from build123d import *

# Parameters (mm, degrees)
EXTRUDE_1_DEPTH            = 10
SKETCH_3_W                 = 250
SKETCH_3_H                 = 25
EXTRUDE_3_DEPTH            = 15
SKETCH_4_W                 = 275.84447974
SKETCH_4_H                 = 25
EXTRUDE_4_DEPTH            = 15
SKETCH_10_W                = 250
SKETCH_10_H                = 30
EXTRUDE_5_DEPTH            = 15
SKETCH_11_W                = 275.84447974
SKETCH_11_H                = 30
EXTRUDE_6_DEPTH            = 15
HOLE_WIZARD_M5_1_D         = 4.2
HOLE_WIZARD_M5_1_DEPTH     = 15
PATTERN_LINEAR_1_COUNT     = 5
PATTERN_LINEAR_1_PITCH     = 50
MIRROR_1_COPY_1_D          = 4.2
MIRROR_1_COPY_1_DEPTH      = 15
MIRROR_1_COPY_2_D          = 4.2
MIRROR_1_COPY_2_DEPTH      = 15
MIRROR_1_COPY_3_D          = 4.2
MIRROR_1_COPY_3_DEPTH      = 15
MIRROR_1_COPY_4_D          = 4.2
MIRROR_1_COPY_4_DEPTH      = 15
HOLE_WIZARD_M5_2_D         = 4.2
PATTERN_START              = 218.95644092
PATTERN_LINEAR_2_OUTLINE_R = 2.1
PATTERN_LINEAR_2_DEPTH     = 15
HOLE_WIZARD_M5_3_D         = 4.2
PATTERN_LINEAR_3_OUTLINE_R = 2.1
PATTERN_LINEAR_3_DEPTH     = 15


# Read off the part's stored shape, not the designer's step: 阵列(线性)2, 阵列(线性)3
with BuildPart() as part:
    # 草图1 → 凸台-拉伸1 (new body)
    with BuildSketch(Plane.XY):
        Polygon((-125.313283208, 0), (124.686716792, 0), (124.686716792, 200), (-125.313283208, 316.576914539), align=None)
        Polygon((-110.313283208, 24.592855818), (-110.313283208, 280.944896886), (14.053831361, 123.772207379), (-107.63654934, 26.72747742), align=None, mode=Mode.SUBTRACT)
        Polygon((23.361623829, 112.009204107), (100.122763689, 15), (-98.284208811, 15), align=None, mode=Mode.SUBTRACT)
        Polygon((109.686716792, 180.85109027), (109.686716792, 27.086733996), (35.089185859, 121.36161211), align=None, mode=Mode.SUBTRACT)
        Polygon((-95.156980934, 285.964131062), (102.096111819, 193.983503317), (100.334376264, 192.57856769), (25.781393391, 133.124615382), align=None, mode=Mode.SUBTRACT)
    extrude(amount=EXTRUDE_1_DEPTH)

    # 草图3 → 凸台-拉伸3 (add)
    with BuildSketch(Plane.XZ):
        with Locations((-0.313283208, 5)):
            Rectangle(SKETCH_3_W, SKETCH_3_H)
    extrude(amount=-EXTRUDE_3_DEPTH)

    # 草图4 → 凸台-拉伸4 (add)
    with BuildSketch(Plane(origin=(98.874264385, 212.036544233, 0), x_dir=(0.9063077870366497, -0.4226182617407002, 0), z_dir=(0.42261826174070016, 0.9063077870366496, 0))):
        with Locations((-109.44134985, -5)):
            Rectangle(SKETCH_4_W, SKETCH_4_H)
    extrude(amount=-EXTRUDE_4_DEPTH)

    # 草图10 → 凸台-拉伸5 (add)
    with BuildSketch(Plane.XZ):
        with Locations((-0.313283208, 32.5)):
            Rectangle(SKETCH_10_W, SKETCH_10_H)
        with Locations((-0.313283208, -22.5)):
            Rectangle(SKETCH_10_W, SKETCH_10_H)
    extrude(amount=-EXTRUDE_5_DEPTH)

    # 草图11 → 凸台-拉伸6 (add)
    with BuildSketch(Plane(origin=(98.874264385, 212.036544233, 0), x_dir=(0.9063077870366497, -0.4226182617407002, 0), z_dir=(0.42261826174070016, 0.9063077870366496, 0))):
        with Locations((-109.44134985, 22.5)):
            Rectangle(SKETCH_11_W, SKETCH_11_H)
        with Locations((-109.44134985, -32.5)):
            Rectangle(SKETCH_11_W, SKETCH_11_H)
    extrude(amount=-EXTRUDE_6_DEPTH)

    # M5 螺纹孔1
    with Locations(Plane(origin=(-100.313283208, 15, 32.5), x_dir=(0, 0, 1), z_dir=(0, 1, 0))):
        with Locations((0, 0)):
            hole_wizard_m5_1 = Hole(HOLE_WIZARD_M5_1_D / 2, depth=HOLE_WIZARD_M5_1_DEPTH)

    # 阵列(线性)1: M5 螺纹孔1 ×5
    with Locations(*[(i * PATTERN_LINEAR_1_PITCH, 0, 0) for i in range(1, PATTERN_LINEAR_1_COUNT)]):
        add(hole_wizard_m5_1, mode=Mode.SUBTRACT)

    # 镜向1: M5 螺纹孔1 across plane
    add(hole_wizard_m5_1.mirror(Plane(origin=(0, 0, 5), x_dir=(1, 0, 0), z_dir=(0, 0, -1))), mode=Mode.SUBTRACT)

    # 镜向1 copy 1
    with Locations(Plane(origin=(-50.313283208, 15, -22.5), x_dir=(0, 0, -1), z_dir=(0, 1, 0))):
        with Locations((0, 0)):
            Hole(MIRROR_1_COPY_1_D / 2, depth=MIRROR_1_COPY_1_DEPTH)

    # 镜向1 copy 2
    with Locations(Plane(origin=(-0.313283208, 15, -22.5), x_dir=(0, 0, -1), z_dir=(0, 1, 0))):
        with Locations((0, 0)):
            Hole(MIRROR_1_COPY_2_D / 2, depth=MIRROR_1_COPY_2_DEPTH)

    # 镜向1 copy 3
    with Locations(Plane(origin=(49.686716792, 15, -22.5), x_dir=(0, 0, -1), z_dir=(0, 1, 0))):
        with Locations((0, 0)):
            Hole(MIRROR_1_COPY_3_D / 2, depth=MIRROR_1_COPY_3_DEPTH)

    # 镜向1 copy 4
    with Locations(Plane(origin=(99.686716792, 15, -22.5), x_dir=(0, 0, -1), z_dir=(0, 1, 0))):
        with Locations((0, 0)):
            Hole(MIRROR_1_COPY_4_D / 2, depth=MIRROR_1_COPY_4_DEPTH)

    # M5 螺纹孔2 (through all)
    with Locations(Plane(origin=(-90.944061912, 300.550283443, -22.5), x_dir=(0.906307787037, -0.422618261741, 0), z_dir=(0.422618261741, 0.906307787037, 0))):
        with Locations((0, 0)):
            Hole(HOLE_WIZARD_M5_2_D / 2)

    # 阵列(线性)2 outline → 阵列(线性)2 (cut)
    with BuildSketch(Plane(origin=(0, 0, 0), x_dir=(0.9063077870366497, -0.42261826174069983, 0), z_dir=(0.4226182617406999, 0.9063077870366498, 0)).offset(PATTERN_START)):
        with Locations((-159.44134985, 22.5)):
            Circle(PATTERN_LINEAR_2_OUTLINE_R)
        with Locations((-109.44134985, 22.5)):
            Circle(PATTERN_LINEAR_2_OUTLINE_R)
        with Locations((-59.44134985, 22.5)):
            Circle(PATTERN_LINEAR_2_OUTLINE_R)
        with Locations((-9.44134985, 22.5)):
            Circle(PATTERN_LINEAR_2_OUTLINE_R)
    extrude(amount=PATTERN_LINEAR_2_DEPTH, mode=Mode.SUBTRACT)

    # M5 螺纹孔3 (through all)
    with Locations(Plane(origin=(-90.944061912, 300.550283443, 32.5), x_dir=(0.906307787037, -0.422618261741, 0), z_dir=(0.422618261741, 0.906307787037, 0))):
        with Locations((0, 0)):
            Hole(HOLE_WIZARD_M5_3_D / 2)

    # 阵列(线性)3 outline → 阵列(线性)3 (cut)
    with BuildSketch(Plane(origin=(0, 0, 0), x_dir=(0.9063077870366497, -0.42261826174069983, 0), z_dir=(0.4226182617406999, 0.9063077870366498, 0)).offset(PATTERN_START)):
        with Locations((-159.44134985, -32.5)):
            Circle(PATTERN_LINEAR_3_OUTLINE_R)
        with Locations((-109.44134985, -32.5)):
            Circle(PATTERN_LINEAR_3_OUTLINE_R)
        with Locations((-59.44134985, -32.5)):
            Circle(PATTERN_LINEAR_3_OUTLINE_R)
        with Locations((-9.44134985, -32.5)):
            Circle(PATTERN_LINEAR_3_OUTLINE_R)
    extrude(amount=PATTERN_LINEAR_3_DEPTH, mode=Mode.SUBTRACT)


solid = part.part
Work out the finished part from the listing and answer in its coordinate system (mm). A direction names the side the tool comes from. Give positions to 0.01 mm unless a question says otherwise; leave off trailing zeros. Order: outer loops, then holes, each group sorted by start corner. A loop starts at its lowest first (then second) coordinate and runs counter-clockwise, first axis right, second up. Notation, with made-up numbers: (9, -33) -> (36, -33) arc R18 cw to (36, -6) -> close; hole circle Ø7 at (-1, 14.25). An arc over 180 degrees is marked (long way). Answer as a JSON object with one key per item and string values. Group by question number.
1. A tool of negligible diameter and unlimited length cuts with its end or side. For faces 1 (the flat face through (-2, 7, 47.5)), 2 (the flat face through (-33.84, 208.47, 4.93)), 3 (the flat face through (121.561, 193.298, -18.487)), from which of +Z, -Z, +X, -X, +Y, -Y can it reach the whole face along a straight path? Write none if from no direction.
2. Consider line 1 along X through (y, z) = (9, 32); line 2 along X through (y, z) = (11.75, 32.5); line 3 along X through (y, z) = (72.5, 1.5). Determine where each line is inside the solid, lowest interval first. Write a range as [from, to].
3. The mould has two halves that part along X. Classify faces 4 (the flat face through (109.687, 105, 5)), 5 (the flat face through (124.687, 62, 5)), 6 (the flat face through (-2, 0, 6)): released by +X, released by -X, zero draft, split by the parting line, or undercut.
4. Section A-A on z = -10 is taken. Determine the outline of the cut face in (x, y).
5. Section B-B on y = 158 is taken. Determine the outline of the cut face in (x, z), plus the area to 3 significant figures.
6. Section C-C on x = -24.5 is taken. Determine the outline of the cut face in (y, z).
7. Flat-ended cylindrical pins translate along their axes: pin 1 Ø3.5 at (x, z) = (99.69, 32.5) entering from -Y; pin 2 Ø1.5 at (x, z) = (-85, 22) entering from +Y; pin 3 Ø1.5 at (y, z) = (208.5, -2.5) entering from -X. Find the tip coordinate at first contact, or state that the pin passes through.
Result sheet:
{
 "1": {"face 1": "+Z, +X, -X, +Y, -Y", "face 2": "+Z, -Z", "face 3": "-Z, +X"},
 "2": {"line 1": "x = [-125.31, -102.35], [-98.27, -52.35], [-48.27, -2.35], [1.73, 47.65], [51.73, 97.65], [101.73, 124.69]", "line 2": "x = [-125.31, -102.41], [-98.21, -52.41], [-48.21, -2.41], [1.79, 47.59], [51.79, 97.59], [101.79, 124.69]", "line 3": "x = [-125.31, -110.31], [-50.24, -26.18], [54.62, 73.75], [109.69, 124.69]"},
 "3": {"face 4": "undercut", "face 5": "released by +X", "face 6": "zero draft"},
 "4": {"outline": "(-131.65, 302.98) -> (118.35, 186.41) -> (124.69, 200) -> (-125.31, 316.58) -> close; (-125.31, 0) -> (124.69, 0) -> (124.69, 15) -> (-125.31, 15) -> close"},
 "5": {"outline": "(-125.31, 0) -> (-110.31, 0) -> (-110.31, 10) -> (-125.31, 10) -> close; (-13.03, 0) -> (6.1, 0) -> (6.1, 10) -> (-13.03, 10) -> close; (56.97, 0) -> (81.03, 0) -> (81.03, 10) -> (56.97, 10) -> close; (109.69, 0) -> (124.69, 0) -> (124.69, 10) -> (109.69, 10) -> close", "area": "732 mm^2"},
 "6": {"outline": "(0, -37.5) -> (15, -37.5) -> (15, 47.5) -> (0, 47.5) -> close; (73.84, 0) -> (93.03, 0) -> (93.03, 10) -> (73.84, 10) -> close; (172.5, 0) -> (196.67, 0) -> (196.67, 10) -> (172.5, 10) -> close; (253.02, -37.5) -> (269.57, -37.5) -> (269.57, 47.5) -> (253.02, 47.5) -> close"},
 "7": {"pin 1": "stops at y = 194.29", "pin 2": "stops at y = 298.13", "pin 3": "stops at x = 69.36"}
}
